from build123d import *

# Parameters (mm, degrees)
POCKET_DEPTH            = 3
POLARPATTERN001_COUNT   = 5
SKETCH007_R             = 1.5
POCKET001_DEPTH         = 5
POCKET001_DEPTH_BACK    = 100
SKETCH008_W             = 18.264466
SKETCH008_H             = 4.2
SKETCH008_R             = 1
PAD004_DEPTH            = 1.2
POLARPATTERN002_COUNT   = 4
BODY003_PLACEMENT_ANGLE = 180


with BuildPart() as part:
    # Sketch005 → Revolution (revolve)
    with BuildSketch(Plane.YZ):
        Polygon((0, 15.3), (2.75, 15.3), (2.75, 13.78), (4.25, 13.78), (4.25, 10.28), (3, 10.28), (3, 7.65), (12.5, 7.65), (13.8, 5.05), (13.8, -5.05), (12.5, -7.65), (3, -7.65), (3, -8.15), (1.5, -8.15), (1.5, -9.15), (0, -9.15), align=None)
    revolve(axis=Axis((0, 0, 0), (0, 0, 1)))

    # Sketch006 (on Face7 of Revolution) → Pocket (cut)
    with BuildSketch(Plane(origin=(0, 0, 7.65), x_dir=(0, -1, 0), z_dir=(0, 0, 1))):
        with BuildLine():
            add(Edge.make_bspline(
                [(-9.307214, 15.452806), (0, 1.064655), (9.307214, 15.452806), (-9.307214, 15.452806)],
                knots=[0, 0, 0, 0, 1, 1, 1, 1], degree=3, weights=[1, 11.84332, 40.102275, 1]))
        make_face()
    pocket = extrude(amount=-POCKET_DEPTH, mode=Mode.SUBTRACT)

    # PolarPattern001: Pocket ×5 about axis
    polarpattern001_axis = Axis((0, 0, 7.65), (0, 0, 1))
    for i in range(1, POLARPATTERN001_COUNT):
        add(pocket.rotate(polarpattern001_axis, i * 360 / POLARPATTERN001_COUNT), mode=Mode.SUBTRACT)

    # Sketch007 → Pocket001 (cut, two sides)
    with BuildSketch(Plane.YZ) as pocket001_sk:
        with Locations((0, 12.025208)):
            Circle(SKETCH007_R)
    extrude(amount=-POCKET001_DEPTH, mode=Mode.SUBTRACT)
    extrude(pocket001_sk.sketch, amount=POCKET001_DEPTH_BACK, mode=Mode.SUBTRACT)

    # Sketch008 (on Face26 of Pocket001) → Pad004 (join)
    with BuildSketch(Plane.YX.offset(7.65)):
        with Locations((8.367767, 0)):
            Rectangle(SKETCH008_W, SKETCH008_H)
        with Locations((15.5, 0)):
            Circle(SKETCH008_R, mode=Mode.SUBTRACT)
    pad004 = extrude(amount=-PAD004_DEPTH)

    # PolarPattern002: Pad004 ×4 about axis
    polarpattern002_axis = Axis((0, 0, -7.65), (0, 0, -1))
    for i in range(1, POLARPATTERN002_COUNT):
        add(pad004.rotate(polarpattern002_axis, i * 360 / POLARPATTERN002_COUNT))


with BuildPart() as part_1:
    # Body003 placement: moved
    add(part.part.moved(Location((0, 66, 15.5))).rotate(Axis((0, 66, 15.5), (0, 1, 0)), BODY003_PLACEMENT_ANGLE))


solid = part_1.part
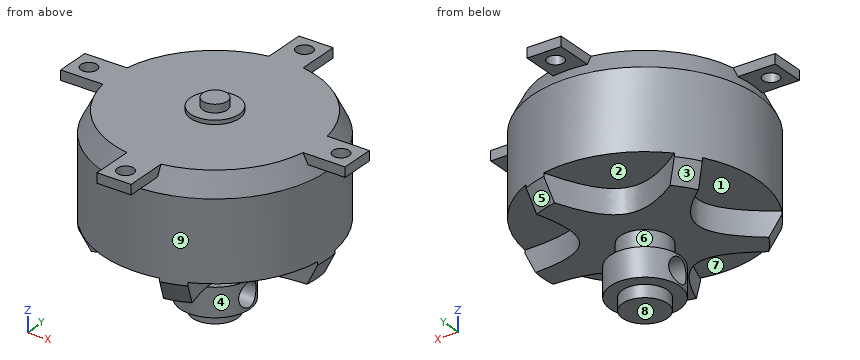
Read the model definition and answer for the solid it produces. Units are mm, in the model's axes. Face numbers are marked on the shaded views. A direction names the side the tool comes from. Round coordinates to 2 decimals unless told otherwise and drop trailing zeros. Loops run counter-clockwise (first coordinate to the right, second up) from the corner with the lowest first, then second, coordinate; pieces in that order, holes last. Notation, with made-up numbers: (6, -30) - (48, -30) arc R28 ccw to (48, 2) - close; hole circle Ø1 at (-8, 89.25). An arc over 180 degrees is marked (long way). One line per question, with ' | ' between items. Start each with the question number.
Q1. Section C-C on x = 0 is taken. Count the separate pieces of the cut face and the enclosed holes in it, plus the area to 3 significant figures.
Q2. Flat-ended cylindrical pins translate along their axes: pin 1 (2.5 mm diameter, centred on x = 0, y = 81.5, fed in from -Z); pin 2 (6 mm diameter, centred on x = -1, y = 58, fed in from -Z); pin 3 (8 mm diameter, centred on x = 12, y = 60.5, fed in from +Z). Find the tip coordinate at first contact, or state that the pin passes through.
Q3. For the marked faces 5, 6, 7, 8 and 9, determine the directions among +Z, -Z, +X, -X, +Y, -Y from which every point of the face is accessible in a straight line to the end or side of a thin tool.
Q4. Section B-B on x = -15.5 is taken. Give the vertices of the cut face in (y, z), plus the area to 3 significant figures.
Q5. Find the intervals of material crossed by L1, parallel to Y at x = 0, z = 22.35; L2, parallel to X at y = 66, z = 22.9; L3, parallel to X at y = 50.5, z = 22.35, in increasing order.
Q6. Section A-A on y = 81.5 is taken. Give the vertices of the cut face in (x, z), plus the area to 3 significant figures.
Q7. Section D-D on z = 4.5 is taken. Give the vertices of the cut face in (x, y).
Q8. For a pull along Y with two mould halves and no side action, classify the marked faces 1, 2, 3 and 4 as +Y half, -Y half, draft (parallel to the pull), parting line (faces both ways), or undercut.
Established:
1) separate pieces: 3 | enclosed holes: 1 | area: 441 mm²
2) pin 1: z = 21.95 | pin 2: z = 7.85 | pin 3: z = 23.15
3) face 5: -Z, +X, +Y | face 6: none | face 7: -Z, -Y | face 8: -Z, +X, -X, +Y, -Y | face 9: -Z
4) outline: (63.9, 21.95) - (65, 21.95) - (65, 23.15) - (63.9, 23.15) - close; (67, 21.95) - (68.1, 21.95) - (68.1, 23.15) - (67, 23.15) - close | area: 2.64 mm²
5) L1: 48.5 to 49.5, 51.5 to 80.5, 82.5 to 83.5 | L2: -17.5 to -16.5, -14.5 to 14.5, 16.5 to 17.5 | L3: -2.1 to -1, 1 to 2.1
6) outline: (-2.1, 21.95) - (-1, 21.95) - (-1, 23.15) - (-2.1, 23.15) - close; (1, 21.95) - (2.1, 21.95) - (2.1, 23.15) - (1, 23.15) - close | area: 2.64 mm²
7) outline: (-4.11, 64.91) arc R4.25 ccw to (4.11, 64.91) - close; (-4.11, 67.09) - (4.11, 67.09) arc R4.25 ccw to start
8) face 1: undercut | face 2: draft | face 3: +Y half | face 4: parting line
